```python
from build123d import *

# Parameters (mm, degrees)
SALIENTE_EXTRUIR1_DEPTH = 590
CROQUIS2_W              = 823.0000000000001
CROQUIS2_H              = 598.4
CORTAR_EXTRUIR1_DEPTH   = 1000
CORTAR_EXTRUIR2_DEPTH   = 1000
CORTAR_EXTRUIR3_DEPTH   = 200
REDONDEO1_R             = 6
REDONDEO2_R             = 6
REDONDEO3_R             = 6


with BuildPart() as part:
    # Croquis1 → Saliente-Extruir1 (new body)
    with BuildSketch(Plane.XY):
        Polygon((0, 0), (950, 0), (950.0000000000001, -700), (8.573e-14, -700), align=None)
    extrude(amount=SALIENTE_EXTRUIR1_DEPTH)

    # Croquis2 → Cortar-Extruir1 (cut)
    with BuildSketch(Plane.XY.offset(590)):
        with Locations((475.00000000000006, -400.8)):
            Rectangle(CROQUIS2_W, CROQUIS2_H)
    extrude(amount=-CORTAR_EXTRUIR1_DEPTH, mode=Mode.SUBTRACT)

    # Croquis3 → Cortar-Extruir2 (cut)
    with BuildSketch(Plane(origin=(950, 1.5067e-13, 0), x_dir=(0, 0, -1), z_dir=(1, 1.6e-16, 0))):
        Polygon((-526.5, -101.60000000000014), (-63.5, -101.60000000000014), (-63.499999999999886, -700.0000000000001), (-526.4999999999999, -700.0000000000001), align=None)
    extrude(amount=-CORTAR_EXTRUIR2_DEPTH, mode=Mode.SUBTRACT)

    # Croquis4 → Cortar-Extruir3 (cut)
    with BuildSketch(Plane(origin=(0, 0, 0), x_dir=(1, 0, 0), z_dir=(0, 1, 0))):
        Polygon((4.857e-14, -63.5), (320.00000000000006, -63.5), (320.0000000000001, -526.5), (5.67e-14, -526.5), align=None)
        Polygon((950, -63.5), (540, -63.50000000000004), (540.0000000000001, -526.4999999999999), (950.0000000000001, -526.4999999999999), align=None)
    extrude(amount=-CORTAR_EXTRUIR3_DEPTH, mode=Mode.SUBTRACT)

    # Redondeo1
    redondeo1_edges = [part.edges().sort_by_distance(p)[0] for p in [
        (0, 0, 31.75),
        (0, 0, 558.25),
        (950, 0, 558.25),
        (950, 0, 31.75),
    ]]
    fillet(redondeo1_edges, radius=REDONDEO1_R)

    # Redondeo2
    redondeo2_edges = [part.edges().sort_by_distance(p)[0] for p in [
        (320.0000000000001, 0, 295),
        (540, 0, 294.99999999999994),
    ]]
    fillet(redondeo2_edges, radius=REDONDEO2_R)

    # Redondeo3
    redondeo3_edges = [part.edges().sort_by_distance(p)[0] for p in [
        (950.0000000000001, -353, 590),
        (948.2426406871193, -1.7573593128807152, 590),
        (4.323e-14, -353, 590),
        (1.7573593128807161, -1.7573593128807143, 590),
        (950.0000000000001, -353, 0),
        (948.2426406871193, -1.7573593128807152, 0),
        (4.323e-14, -353, 0),
        (1.7573593128807161, -1.7573593128807143, 0),
        (950.0000000000001, -353, 526.4999999999999),
        (948.2426406871193, -1.7573593128807152, 526.4999999999999),
        (7.839e-14, -353, 526.4999999999999),
        (1.7573593128807161, -1.7573593128807143, 526.5),
        (7.436e-14, -353, 63.49999999999994),
        (1.7573593128807161, -1.7573593128807143, 63.5),
        (950.0000000000001, -353, 63.49999999999994),
        (948.2426406871193, -1.7573593128807152, 63.5),
        (475, 0, 590),
        (475, 0, 0),
        (739, 0, 526.4999999999999),
        (166.00000000000006, 4.4e-16, 526.5),
        (166.00000000000003, 4.4e-16, 63.5),
        (739, 0, 63.50000000000002),
    ]]
    fillet(redondeo3_edges, radius=REDONDEO3_R)


solid = part.part
```
The listing builds one solid part. Answer for the finished solid, in the listing's coordinates (mm). A direction names the side the tool comes from. Give positions to 0.01 mm unless a question says otherwise; leave off trailing zeros. Order: outer loops, then holes, each group sorted by start corner. A loop starts at its lowest first (then second) coordinate and runs counter-clockwise, first axis right, second up. Notation, with made-up numbers: (77.25, 23.25) - (107.25, 23.25) arc R16 cw to (107.25, 48.25) - close; hole circle Ø6 at (-0.75, -33.75). An arc over 180 degrees is marked (long way). Answer in a Markdown table with one row per item. Add a question column.
Q1. The part is cut by section A-A (x = 611). Determine the outline of the cut face in (y, z), then the cut area to 3 significant figures.
Q2. The part is cut by section B-B (y = -433). Determine the outline of the cut face in (x, z), then the cut area to 3 significant figures.
Q3. For a pull along Z with two mould halves and no side action, classify faces 4 (the flat face through (477, -94, 590)), 5 (the flat face through (919, -700, 558)), 6 (the flat face through (540, -53, 292)) as released by +Z, released by -Z, zero draft, split by the parting line, or undercut.
Q4. Which of the six approach directions +Z, -Z, +X, -X, +Y, -Y give full straight-line access (tool end or side, diameter ignored) to faces 1 (the flat face through (893, -197, 63.5)), 2 (the flat face through (320, -53, 292)), 3 (the flat face through (63.5, -405, 32))?
Q5. Find the intervals of material crossed by line 1 along X through (y, z) = (-572.5, 35); line 2 along Z through (x, y) = (185, -40); line 3 along Y through (x, z) = (393.5, 536), in increasing order. Write a range as [from, to].
Q6. The part is cut by section D-D (z = 381.5). Determine the outline of the cut face in (x, y).
Q7. The part is cut by section C-C (y = -55). Determine the outline of the cut face in (x, z), then the cut area to 3 significant figures.
Determined:
| question | item | result |
|---|---|---|
| 1 | outline | (-101.6, 0) - (-6, 0) arc R6 ccw to (0, 6) - (0, 57.5) arc R6 ccw to (-6, 63.5) - (-101.6, 63.5) - close; (-101.6, 526.5) - (-6, 526.5) arc R6 ccw to (0, 532.5) - (0, 584) arc R6 ccw to (-6, 590) - (-101.6, 590) - close |
| 1 | area | 12,900 mm² |
| 2 | outline | (0, 6) arc R6 ccw to (6, 0) - (63.5, 0) - (63.5, 63.5) - (6, 63.5) arc R6 ccw to (0, 57.5) - close; (0, 532.5) arc R6 ccw to (6, 526.5) - (63.5, 526.5) - (63.5, 590) - (6, 590) arc R6 ccw to (0, 584) - close; (886.5, 0) - (944, 0) arc R6 ccw to (950, 6) - (950, 57.5) arc R6 ccw to (944, 63.5) - (886.5, 63.5) - close; (886.5, 526.5) - (944, 526.5) arc R6 ccw to (950, 532.5) - (950, 584) arc R6 ccw to (944, 590) - (886.5, 590) - close |
| 2 | area | 16,100 mm² |
| 3 | face 4 | released by +Z |
| 3 | face 5 | zero draft |
| 3 | face 6 | undercut |
| 4 | face 1 | +X, +Y, -Y |
| 4 | face 2 | -X, +Y, -Y |
| 4 | face 3 | +Z, -Z, -Y |
| 5 | line 1 | x = [0, 63.5], [886.5, 950] |
| 5 | line 2 | z = [0, 63.5], [526.5, 590] |
| 5 | line 3 | y = [-101.6, 0] |
| 6 | outline | (320, -101.6) - (540, -101.6) - (540, -6) arc R6 ccw to (534, 0) - (326, 0) arc R6 ccw to (320, -6) - close |
| 7 | outline | (0, 6) arc R6 ccw to (6, 0) - (944, 0) arc R6 ccw to (950, 6) - (950, 57.5) arc R6 ccw to (944, 63.5) - (540, 63.5) - (540, 526.5) - (944, 526.5) arc R6 ccw to (950, 532.5) - (950, 584) arc R6 ccw to (944, 590) - (6, 590) arc R6 ccw to (0, 584) - (0, 532.5) arc R6 ccw to (6, 526.5) - (320, 526.5) - (320, 63.5) - (6, 63.5) arc R6 ccw to (0, 57.5) - close |
| 7 | area | 222,000 mm² |
